```python
from build123d import *

# Parameters (mm, degrees)
SKETCH1_W           = 1500.847015591
SKETCH1_H           = 50.8
BOSS_EXTRUDE2_DEPTH = 609.6
SKETCH3_W           = 1473.2
SKETCH3_H           = 558.8
BOSS_EXTRUDE4_DEPTH = 200
SKETCH4_R           = 50
BOSS_EXTRUDE5_DEPTH = 50
SKETCH5_R           = 40
CUT_EXTRUDE3_DEPTH  = 200
BOSS_EXTRUDE6_DEPTH = 50


with BuildPart() as part:
    # Sketch1 → Boss-Extrude2 (new body)
    with BuildSketch(Plane.XY):
        Polygon((0, 0), (1500.847015591, 0), (1500.847015591, 264.639822764), align=None)
        with Locations((750.423507796, -25.4)):
            Rectangle(SKETCH1_W, SKETCH1_H)
    extrude(amount=BOSS_EXTRUDE2_DEPTH)

    # Sketch3 → Boss-Extrude4 (add)
    with BuildSketch(Plane(origin=(0, 0, 0), x_dir=(0.9848077530122079, 0.17364817766693136, 0), z_dir=(-0.17364817766693136, 0.9848077530122079, 0))):
        Polygon((1524, 0), (0, 0), (0, -25.4), (0, -609.6), (1524, -609.6), align=None)
        with Locations((762, -304.8)):
            Rectangle(SKETCH3_W, SKETCH3_H, mode=Mode.SUBTRACT)
    extrude(amount=BOSS_EXTRUDE4_DEPTH)

    # Sketch4 → Boss-Extrude5 (add)
    with BuildSketch(Plane(origin=(0, 0, 0), x_dir=(0.9848077530122079, 0.17364817766693136, 0), z_dir=(-0.17364817766693136, 0.9848077530122079, 0))):
        with Locations(Location((125.4, -304.8, 0), (0, 0, 180))):
            Circle(SKETCH4_R)
    extrude(amount=BOSS_EXTRUDE5_DEPTH)

    # Sketch5 → Cut-Extrude3 (cut)
    with BuildSketch(Plane(origin=(-8.682408883, 49.240387651, 0), x_dir=(0.9848077530122079, 0.17364817766693136, 0), z_dir=(-0.17364817766693136, 0.9848077530122079, 0))):
        with Locations(Location((125.4, -304.8, 0), (0, 0, 180))):
            Circle(SKETCH5_R)
    extrude(amount=-CUT_EXTRUDE3_DEPTH, mode=Mode.SUBTRACT)

    # Sketch6 → Boss-Extrude6 (add)
    with BuildSketch(Plane(origin=(0, -50.8, 0), x_dir=(-1, 0, 0), z_dir=(0, -1, 0))):
        Polygon((-350, 0), (-350, -609.6), (-300, -609.6), (-300, -304.8), (-300, 0), align=None)
        Polygon((-1200.847015591, 0), (-1200.847015591, -304.8), (-1200.847015591, -609.6), (-1150.847015591, -609.6), (-1150.847015591, 0), align=None)
    extrude(amount=BOSS_EXTRUDE6_DEPTH)


solid = part.part
```
Work out the finished part from the listing and answer in its coordinate system (mm). A direction names the side the tool comes from. Coordinates: 2 decimals unless noted, no trailing zeros. Loops run counter-clockwise (first coordinate to the right, second up) from the corner with the lowest first, then second, coordinate; pieces in that order, holes last. Notation, with made-up numbers: M -8.5,40.25 L 5.5,40.25 A6 ccw 5.5,46.25 Z; hole C 52.25,-2 d6. An arc over 180 degrees is marked long. Use CSV: the item, a comma, the result in double quotes. Start each with the question number.
(1) Find section B-B, the plane y = 292. Give the vertices of the cut face in (x, z).
(2) Find section D-D, the plane x = 229. Give the vertices of the cut face in (y, z), then the cut area to 3 significant figures.
(3) Find section C-C, the plane z = 465. Give the vertices of the cut face in (x, y).
(4) Find section A-A, the plane z = 283.5. Give the vertices of the cut face in (x, y), then the cut area to 3 significant figures.
(5) For a pull along Z with two mould halves and no side action, classify faces 1 (the face through (736, 128, 609.6)), 2 (the face through (129.89, 47.93, 255.99)), 3 (the face through (181, -50.8, 301)) as +Z half, -Z half, draft (parallel to the pull), parting line (faces both ways), or undercut.
(6) Given pin 1 Ø25 at (y, z) = (-84.5, 455) entering from -X; pin 2 Ø1.5 at (x, z) = (1326, 223) entering from +Y; pin 3 Ø4 at (y, z) = (337.5, 258) entering from +X, each flat-ended and moving along its own axis, determine where each tip first touches the part or whether it passes through.
(7) For faces 4 (the face through (350, -75, 301)), 5 (the face through (136.927, 74.915, 338.367)), 6 (the face through (1200.847, -75, 301)), determine the directions among +Z, -Z, +X, -X, +Y, -Y from which every point of the face is accessible in a straight line to the end or side of a thin tool.
(8) Consider line 1 (Z direction, x = 1130.5, y = 365); line 2 (X direction, y = -70, z = 218.5); line 3 (Y direction, x = 146, z = 205). Determine where each line is inside the solid, lowest interval first.
Recorded:
1,outline,"M 504.26,0 L 1496.02,0 L 1496.02,609.6 L 504.26,609.6 L 504.26,584.2 L 1470.23,584.2 L 1470.23,25.4 L 504.26,25.4 Z"
2,outline,"M -50.8,0 L 243.46,0 L 243.46,25.4 L 40.38,25.4 L 40.38,584.2 L 243.46,584.2 L 243.46,609.6 L -50.8,609.6 Z"
2,area,"65,900 mm^2"
3,outline,"M -34.73,196.96 L 0,0 L 0,-50.8 L 300,-50.8 L 300,-100.8 L 350,-100.8 L 350,-50.8 L 1150.85,-50.8 L 1150.85,-100.8 L 1200.85,-100.8 L 1200.85,-50.8 L 1500.85,-50.8 L 1500.85,264.64 L 1466.12,461.6 L 1441.1,457.19 L 1475.83,260.23 L 25.01,4.41 L -9.72,201.37 Z"
4,outline,"M -34.73,196.96 L 0,0 L 0,-50.8 L 101.91,-50.8 L 81.47,65.14 L 70.26,63.16 L 78.95,13.92 L 25.01,4.41 L -9.72,201.37 Z; M 148.16,76.9 L 170.67,-50.8 L 300,-50.8 L 300,-100.8 L 350,-100.8 L 350,-50.8 L 1150.85,-50.8 L 1150.85,-100.8 L 1200.85,-100.8 L 1200.85,-50.8 L 1500.85,-50.8 L 1500.85,264.64 L 1466.12,461.6 L 1441.1,457.19 L 1475.83,260.23 L 168.04,29.63 L 159.36,78.87 Z"
4,area,"286,000 mm^2"
5,face 1,"+Z half"
5,face 2,"undercut"
5,face 3,"draft"
6,pin 1,"stops at x = 300"
6,pin 2,"stops at y = 233.94"
6,pin 3,"stops at x = 1488.35"
7,face 4,"+Z, -Z, -Y"
7,face 5,"+Y"
7,face 6,"+Z, -Z, +X, -Y"
8,line 1,"z = 0 to 25.4, 584.2 to 609.6"
8,line 2,"x = 300 to 350, 1150.85 to 1200.85"
8,line 3,"y = -50.8 to 25.74"
